Can you work these out from the model? Positions are in its coordinate system, mm. Coordinates: 2 decimals unless noted, no trailing zeros. Order: outer loops, then holes, each group sorted by start corner. A loop starts at its lowest first (then second) coordinate and runs counter-clockwise, first axis right, second up. Notation, with made-up numbers: M -1.75,67.5 L 19.25,67.5 A18 cw 19.25,102.5 Z; hole C -9.75,-30 d11. An arc over 180 degrees is marked long. Answer as CSV lines item,"result". Start each with the question number.
1. If we section it at C-C (y = 47): List the corners of the cut face in (x, z) for me, plus the area to 3 significant figures.
2. If we mould it in two halves opening along Y, with no side actions, what happens to faces 1 (the face through (29, 25.857, 1)), 2 (the face through (25.664, 53.799, 1.479)), 3 (the face through (55, 30, 3)), 4 (the face through (53.761, 13.445, 1.479))? For each: released by +Y, released by -Y, zero draft, split by the parting line, or undercut.
3. I need wall thicknesses on line 1 along X through (y, z) = (46.5, 0.3); line 2 along X through (y, z) = (14.5, 2.2); line 3 along X through (y, z) = (16, 1.2). Which ranges of each line are inside material? Lowest first, please. Write a range as from..to.
4. Will these pins go through, and if not, where does the flat tip stop? pin 1 (1.5 mm diameter, centred on x = 40.5, z = 2, fed in from +Y); pin 2 (0.9 mm diameter, centred on x = 48, z = 1, fed in from +Y); pin 3 (1.5 mm diameter, centred on x = 29, z = 1.5, fed in from +Y).
5. If we section it at B-B (x = 38.5): List the corners of the cut face in (y, z) for me, plus the area to 3 significant figures.
6. If we section it at A-A (x = 51.5): List the corners of the cut face in (y, z) for me, plus the area to 3 significant figures.
7. If we section it at D-D (x = 30): List the corners of the cut face in (y, z) for me.
```python
from build123d import *

# Parameters (mm, degrees)
MODEL_R             = 1.300000008
MODEL_R_2           = 1.3
MODEL_R_3           = 1.500000002
MODEL_W             = 3
MODEL_H             = 6
MODEL_W_2           = 23
MODEL_H_2           = 12
MODEL_W_3           = 10
MODEL_H_3           = 3
BOSS_EXTRUDE1_DEPTH = 3


with BuildPart() as part:
    # Model → Boss-Extrude1 (new body)
    with BuildSketch(Plane.XY):
        with BuildLine():
            Line((24.95163, 51.857462577), (24.95163, 11.157702759))
            ThreePointArc((24.95163, 11.157702759), (25.830365801, 9.036226784), (27.95183001, 8.157462577))
            Line((27.95183001, 8.157462577), (81.95183001, 8.157462577))
            ThreePointArc((81.95183001, 8.157462577), (84.0730792, 9.036166136), (84.951725641, 11.157438987))
            Line((84.951725641, 11.157438987), (84.95183, 51.857462577))
            ThreePointArc((84.95183, 51.857462577), (84.848554916, 52.637712888), (84.54593, 53.364262577))
            Line((84.54593, 53.364262577), (79.66303, 61.771262577))
            ThreePointArc((79.66303, 61.771262577), (77.874800295, 63.39663974), (75.47683, 63.695562577))
            Line((75.47683, 63.695562577), (27.40633, 54.807462577))
            ThreePointArc((27.40633, 54.807462577), (25.64557658, 53.776308467), (24.95163, 51.857462577))
        make_face()
        with Locations((45.451629992, 52.357462585)):
            Circle(MODEL_R, mode=Mode.SUBTRACT)
        with Locations((45.451829992, 33.357462569)):
            Circle(MODEL_R, mode=Mode.SUBTRACT)
        with Locations((76.20413, 59.762262577)):
            Circle(MODEL_R_2, mode=Mode.SUBTRACT)
        with Locations((54.951729998, 14.357462579)):
            Circle(MODEL_R_3, mode=Mode.SUBTRACT)
        with Locations((29.451829998, 22.357462575)):
            Circle(MODEL_R_3, mode=Mode.SUBTRACT)
        with Locations((80.451829998, 42.357462575)):
            Circle(MODEL_R_3, mode=Mode.SUBTRACT)
        with Locations((29.45183, 28.857462577)):
            Rectangle(MODEL_W, MODEL_H, mode=Mode.SUBTRACT)
        with Locations((45.45183, 42.857462577)):
            Rectangle(MODEL_W_2, MODEL_H_2, mode=Mode.SUBTRACT)
        with Locations((29.45183, 15.857462577)):
            Rectangle(MODEL_W, MODEL_H, mode=Mode.SUBTRACT)
        with Locations((37.45183, 14.357462577)):
            Rectangle(MODEL_W_3, MODEL_H_3, mode=Mode.SUBTRACT)
        with Locations((72.45183, 14.357462577)):
            Rectangle(MODEL_W_3, MODEL_H_3, mode=Mode.SUBTRACT)
        with Locations((80.45183, 35.857462577)):
            Rectangle(MODEL_W, MODEL_H, mode=Mode.SUBTRACT)
        with Locations((80.45183, 48.857462577)):
            Rectangle(MODEL_W, MODEL_H, mode=Mode.SUBTRACT)
    extrude(amount=BOSS_EXTRUDE1_DEPTH)


solid = part.part
```
Solved:
1,outline,"M 24.95,0 L 33.95,0 L 33.95,3 L 24.95,3 Z; M 56.95,0 L 78.95,0 L 78.95,3 L 56.95,3 Z; M 81.95,0 L 84.95,0 L 84.95,3 L 81.95,3 Z"
1,area,"102 mm²"
2,face 1,"undercut"
2,face 2,"released by +Y"
2,face 3,"zero draft"
2,face 4,"undercut"
3,line 1,"24.95..33.95, 56.95..78.95, 81.95..84.95"
3,line 2,"24.95..27.95, 30.95..32.45, 42.45..53.46, 56.44..67.45, 77.45..84.95"
3,line 3,"24.95..27.95, 30.95..84.95"
4,pin 1,"y = 57.37"
4,pin 2,"y = 58.7"
4,pin 3,"y = 55.24"
5,outline,"M 8.16,0 L 12.86,0 L 12.86,3 L 8.16,3 Z; M 15.86,0 L 36.86,0 L 36.86,3 L 15.86,3 Z; M 48.86,0 L 56.86,0 L 56.86,3 L 48.86,3 Z"
5,area,"101 mm²"
6,outline,"M 8.16,0 L 36.86,0 L 36.86,3 L 8.16,3 Z; M 48.86,0 L 59.26,0 L 59.26,3 L 48.86,3 Z"
6,area,"117 mm²"
7,outline,"M 8.16,0 L 12.86,0 L 12.86,3 L 8.16,3 Z; M 18.86,0 L 20.96,0 L 20.96,3 L 18.86,3 Z; M 23.75,0 L 25.86,0 L 25.86,3 L 23.75,3 Z; M 31.86,0 L 55.29,0 L 55.29,3 L 31.86,3 Z"
